Autodesk Inventor part; units mm, degrees
ref_plane "YZ Plane" through (0, 0, 0) normal (1, 0, 0) x (0, 1, 0)
ref_plane "XZ Plane" through (0, 0, 0) normal (0, 1, 0) x (-1, 0, 0)
ref_plane "XY Plane" through (0, 0, 0) normal (0, 0, 1) x (1, 0, 0)
sketch "Sketch1" plane through (0, 0, 0) normal (0, 0, 1) x (1, 0, 0)
  line L0 (0, 0) -> (153, 0)
  line L1 (153, 0) -> (153, 43)
  line L2 (153, 43) -> (0, 43)
  line L3 (0, 43) -> (0, 0)
  dimension "d0" = 43
  dimension "d1" = 153
extrude "Extrusion1" add sketch "Sketch1" along normal blind 6.35
chamfer "Chamfer1" distance 2 angle 45 4 edges at (0, 43, 3.175) (0, 0, 3.175) (153, 43, 3.175) (153, 0, 3.175)
ref_plane "Work Plane1" through (2, 21.5, 0) normal (0, 1, 0) x (1, 0, 0)
ref_plane "Work Plane2" through (76.5, 2, 0) normal (1, 0, 0) x (0, 0, -1)
sketch "Sketch2" plane through (0, 0, 6.35) normal (0, 0, 1) x (1, 0, 0)
  line L0 (137.7, 37.4031) -> (143.5031, 31.6)
  line L1 (149.525, 31.6) -> (143.5031, 31.6)
  line L2 (152.7, 34.775) -> (149.525, 31.6)
  line L3 (152.7, 43.2063) -> (152.7, 34.775)
  line L4 (152.7, 43.2063) -> (0.3, 43.2063)
  line L5 (0.3, 34.775) -> (0.3, 43.2063)
  line L6 (3.475, 31.6) -> (0.3, 34.775)
  line L7 (9.4969, 31.6) -> (3.475, 31.6)
  line L8 (9.4969, 31.6) -> (15.3, 37.4031)
  line L9 (15.3, 37.4031) -> (66.5, 37.4031)
  line L10 (66.5, 37.4031) -> (72.3031, 31.6)
  line L11 (80.6969, 31.6) -> (72.3031, 31.6)
  line L12 (80.6969, 31.6) -> (86.5, 37.4031)
  line L13 (86.5, 37.4031) -> (137.7, 37.4031)
  circle A0 centre (76.5, 37.4031) radius 1.7018
  circle A1 centre (147.7, 37.4031) radius 1.7018
  circle A2 centre (5.3, 37.4031) radius 1.7018
  line L14 (15.27, 5.5969) -> (9.4669, 11.4)
  line L15 (3.445, 11.4) -> (9.4669, 11.4)
  line L16 (0.27, 8.225) -> (3.445, 11.4)
  line L17 (0.27, -0.2063) -> (0.27, 8.225)
  line L18 (0.27, -0.2063) -> (152.67, -0.2063)
  line L19 (152.67, 8.225) -> (152.67, -0.2063)
  line L20 (149.495, 11.4) -> (152.67, 8.225)
  line L21 (143.4731, 11.4) -> (149.495, 11.4)
  line L22 (143.4731, 11.4) -> (137.67, 5.5969)
  line L23 (137.67, 5.5969) -> (86.47, 5.5969)
  line L24 (86.47, 5.5969) -> (80.6669, 11.4)
  line L25 (72.2731, 11.4) -> (80.6669, 11.4)
  line L26 (72.2731, 11.4) -> (66.47, 5.5969)
  line L27 (66.47, 5.5969) -> (15.27, 5.5969)
  circle A3 centre (76.47, 5.5969) radius 1.7018
  circle A4 centre (5.27, 5.5969) radius 1.7018
  circle A5 centre (147.67, 5.5969) radius 1.7018
  point P0 (0, 0)
  point P1 (76.47, 5.5969)
  point P2 (5.27, 5.5969)
  point P3 (147.67, 5.5969)
hole "Hole1" at (147.7, 37.4031, 6.35) at (76.5, 37.4031, 6.35) at (5.3, 37.4031, 6.35) at (5.27, 5.5969, 6.35) at (76.47, 5.5969, 6.35) at (147.67, 5.5969, 6.35) direction (0, 0, -1) diameter 3.4 depth 8 tip angle 118 countersink diameter 6.3 countersink angle 90
properties part number "Rear Armor" material "Polyethylene, High Density"
The listing builds one solid part. Answer for the finished solid, in the listing's coordinates (mm). Give positions to 0.01 mm unless a question says otherwise; leave off trailing zeros. Use a Markdown table: item, result.
1. Find the intervals of material crossed by probe 1 along Y at (x, z) = (5.3, 1); probe 2 along X at (y, z) = (38, 2.75); probe 3 along X at (y, z) = (6, 2.5), in increasing order. Write a range as from..to.
Values follow:
| item | result |
|---|---|
| probe 1 | y = 0..3.9, 7.3..35.7, 39.1..43 |
| probe 2 | x = 0..3.71, 6.89..74.91, 78.09..146.11, 149.29..153 |
| probe 3 | x = 0..3.62, 6.92..74.82, 78.12..146.02, 149.32..153 |
2. Each of these flat-tipped pins is pushed along its axis until it touches: P1, Ø1.5, axis at x = 119, y = 8, coming from the -Z side; P2, Ø4.5, axis at x = 147.67, y = 5.6, coming from the +Z side. Where does it stop, or does it pass through?
Values follow:
| item | result |
|---|---|
| P1 | stops at z = 0 |
| P2 | stops at z = 5.45 |
3. For a pull along Y with two mould halves and no side action, classify faces 1 (the flat face through (0, 22, 3)), 2 (the flat face through (75, 0, 3)), 3 (the cylindrical face through (78.13, 5.97, 2.42)) as released by +Y, released by -Y, zero draft, split by the parting line, or undercut.
Values follow:
| item | result |
|---|---|
| face 1 | zero draft |
| face 2 | released by -Y |
| face 3 | undercut |
